```python
from build123d import *

# Parameters (mm, degrees)
SKETCH2_R           = 2
BOSS_EXTRUDE1_DEPTH = 14
SKETCH7_R           = 12.060749
CUT_EXTRUDE4_DEPTH  = 8
SKETCH8_R           = 2
CUT_EXTRUDE5_DEPTH  = 8
FILLET2_R           = 2
FILLET4_R           = 2
SKETCH10_R          = 4
BOSS_EXTRUDE3_DEPTH = 3
SKETCH13_R          = 4.000853
BOSS_EXTRUDE4_DEPTH = 3
SKETCH15_R          = 2.9
SKETCH15_R_2        = 1.5
BOSS_EXTRUDE5_DEPTH = 9
SKETCH16_R          = 2.9
SKETCH16_R_2        = 1.5
BOSS_EXTRUDE6_DEPTH = 9
CIRPATTERN1_COUNT   = 3


with BuildPart() as part:
    # Sketch2 → Boss-Extrude1 (new body)
    with BuildSketch(Plane.XY):
        with BuildLine():
            Line((-7, 23), (-7, 37))
            Line((-7, 37), (7, 37))
            Line((7, 37), (7, 23))
            ThreePointArc((7, 23), (13.037466, 7.527184), (23.418584, -5.437822))
            Line((23.418584, -5.437822), (35.54294, -12.437822))
            Line((35.54294, -12.437822), (28.54294, -24.562178))
            Line((28.54294, -24.562178), (16.418584, -17.562178))
            ThreePointArc((16.418584, -17.562178), (0, -15.054369), (-16.418584, -17.562178))
            Line((-16.418584, -17.562178), (-28.54294, -24.562178))
            Line((-28.54294, -24.562178), (-35.54294, -12.437822))
            Line((-35.54294, -12.437822), (-23.418584, -5.437822))
            ThreePointArc((-23.418584, -5.437822), (-13.037466, 7.527184), (-7, 23))
        make_face()
        Circle(SKETCH2_R, mode=Mode.SUBTRACT)
    extrude(amount=BOSS_EXTRUDE1_DEPTH)

    # Sketch7 → Cut-Extrude4 (cut)
    with BuildSketch(Plane.XY.offset(14)):
        Circle(SKETCH7_R)
    extrude(amount=-CUT_EXTRUDE4_DEPTH, mode=Mode.SUBTRACT)

    # Sketch8 → Cut-Extrude5 (cut)
    with BuildSketch(Plane.XY.offset(6)):
        with Locations((0, 8)):
            Circle(SKETCH8_R)
        with Locations((6.254652, 4.987918)):
            Circle(SKETCH8_R)
        with Locations((7.799423, -1.780167)):
            Circle(SKETCH8_R)
        with Locations((3.47107, -7.207751)):
            Circle(SKETCH8_R)
        with Locations((-3.47107, -7.207751)):
            Circle(SKETCH8_R)
        with Locations((-7.799423, -1.780167)):
            Circle(SKETCH8_R)
        with Locations((-6.254652, 4.987918)):
            Circle(SKETCH8_R)
    extrude(amount=-CUT_EXTRUDE5_DEPTH, mode=Mode.SUBTRACT)

    # Fillet2
    fillet2_edges = [part.edges().sort_by_distance(p)[0] for p in [
        (32.04294, -18.5, 0),
        (-32.04294, -18.5, 0),
        (0, 37, 0),
        (-32.04294, -18.5, 14),
        (32.04294, -18.5, 14),
        (0, 37, 14),
    ]]
    fillet(fillet2_edges, radius=FILLET2_R)

    # Fillet4
    fillet4_edges = [part.edges().sort_by_distance(p)[0] for p in [
        (7, 29, 0),
        (13.037466, 7.527184, 0),
        (-13.037466, 7.527184, 14),
        (21.614737, -20.562178, 0),
        (0, -15.054369, 0),
        (-28.614737, -8.437822, 0),
        (-13.037466, 7.527184, 0),
        (-28.614737, -8.437822, 14),
        (0, -15.054369, 14),
        (21.614737, -20.562178, 14),
        (13.037466, 7.527184, 14),
        (7, 29, 14),
        (-7, 37, 7),
        (7, 37, 7),
        (-7, 29, 0),
        (-7, 29, 14),
        (-7, 36.414214, 13.414214),
        (-7, 36.414214, 0.585786),
        (28.614737, -8.437822, 0),
        (-21.614737, -20.562178, 0),
        (7, 36.414214, 13.414214),
        (7, 36.414214, 0.585786),
        (-21.614737, -20.562178, 14),
        (28.614737, -8.437822, 14),
        (-28.54294, -24.562178, 7),
        (-35.54294, -12.437822, 7),
        (-28.035634, -24.269285, 13.414214),
        (-28.035634, -24.269285, 0.585786),
        (-35.035634, -12.144929, 13.414214),
        (-35.035634, -12.144929, 0.585786),
        (35.54294, -12.437822, 7),
        (28.54294, -24.562178, 7),
        (35.035634, -12.144929, 13.414214),
        (35.035634, -12.144929, 0.585786),
        (28.035634, -24.269285, 13.414214),
        (28.035634, -24.269285, 0.585786),
    ]]
    fillet(fillet4_edges, radius=FILLET4_R)

    # Sketch10 → Boss-Extrude3 (add)
    with BuildSketch(Plane(origin=(3.5, 6.062178, 0), x_dir=(0.866025403784439, -0.4999999999999995, 0), z_dir=(0.49999999999999944, 0.8660254037844389, 0))):
        with Locations((29.5, -7)):
            Circle(SKETCH10_R)
    boss_extrude3 = extrude(amount=BOSS_EXTRUDE3_DEPTH)

    # Sketch13 → Boss-Extrude4 (add)
    with BuildSketch(Plane(origin=(-3.5, -6.062178, 0), x_dir=(0.8660254037844386, -0.5, 0), z_dir=(-0.5000000000000001, -0.8660254037844387, 0))):
        with Locations(Location((29.5, 7, 0), (0, 0, 180))):
            Circle(SKETCH13_R)
    boss_extrude4 = extrude(amount=BOSS_EXTRUDE4_DEPTH)

    # Sketch15 → Boss-Extrude5 (add)
    with BuildSketch(Plane(origin=(5, 8.660254, 0), x_dir=(0.8660254037844389, -0.4999999999999997, 0), z_dir=(0.4999999999999997, 0.8660254037844389, 0))):
        with Locations(Location((29.5, -7, 0), (0, 0, 180))):
            Circle(SKETCH15_R)
        with Locations(Location((29.5, -7, 0), (0, 0, 180))):
            Circle(SKETCH15_R_2, mode=Mode.SUBTRACT)
    boss_extrude5 = extrude(amount=BOSS_EXTRUDE5_DEPTH)

    # Sketch16 → Boss-Extrude6 (add)
    with BuildSketch(Plane(origin=(-5, -8.660254, 0), x_dir=(0.8660254037844386, -0.4999999999999999, 0), z_dir=(-0.49999999999999994, -0.8660254037844387, 0))):
        with Locations(Location((29.5, 7, 0), (0, 0, 180))):
            Circle(SKETCH16_R)
        with Locations(Location((29.5, 7, 0), (0, 0, 180))):
            Circle(SKETCH16_R_2, mode=Mode.SUBTRACT)
    boss_extrude6 = extrude(amount=BOSS_EXTRUDE6_DEPTH)

    # CirPattern1: Boss-Extrude3, Boss-Extrude4, Boss-Extrude5, Boss-Extrude6 ×3 about axis
    cirpattern1_axis = Axis((0, 0, 0), (0, 0, 1))
    add([boss_extrude3.rotate(cirpattern1_axis, i * 360 / CIRPATTERN1_COUNT) for i in range(1, CIRPATTERN1_COUNT)])
    add([boss_extrude4.rotate(cirpattern1_axis, i * 360 / CIRPATTERN1_COUNT) for i in range(1, CIRPATTERN1_COUNT)])
    add([boss_extrude5.rotate(cirpattern1_axis, i * 360 / CIRPATTERN1_COUNT) for i in range(1, CIRPATTERN1_COUNT)])
    add([boss_extrude6.rotate(cirpattern1_axis, i * 360 / CIRPATTERN1_COUNT) for i in range(1, CIRPATTERN1_COUNT)])


solid = part.part
```
CAD build for the part. Positions are in the model's coordinates, mm. A direction names the side the tool comes from. Round coordinates to 2 decimals unless told otherwise and drop trailing zeros. Loops run counter-clockwise (first coordinate to the right, second up) from the corner with the lowest first, then second, coordinate; pieces in that order, holes last. Notation, with made-up numbers: M -2,8 L 27,8 A20 cw 27,38 Z; hole C 88.5,67.25 d10. An arc over 180 degrees is marked long. Return JSON: item names as keys, results as strings. Group by question number.
(1) Saw through at C-C, the plane y = -28. Give the number of separate pieces and of enclosed holes in the cut face, and give its area (3 significant figures).
(2) Drop flat-ended pins along their axis: P1, Ø3, axis at y = -2.5, z = 4.5, coming from the -X side; P2, Ø3.5, axis at x = 0, y = 0, coming from the +Z side; P3, Ø2.5, axis at y = 29.5, z = 5.5, coming from the +X side; P4, Ø2.5, axis at y = 29.5, z = 7, coming from the -X side. Give the stop position or say it passes through.
(3) Tool access for faces 1 (the cylindrical face through (8.479, 25.684, 5.798)), 2 (the flat face through (-15, -30.6, 5.8)), 3 (the cylindrical face through (21.895, -20.029, 13.43)), 4 (the cylindrical face through (-2.615, -11.774, 10.056)), 5 (the cylindrical face through (-6.43, 28.8, 13.4)): list every direction of +Z, -Z, +X, -X, +Y, -Y with a clear straight run to the whole face (end or side of a thin tool).
(4) Saw through at A-A, the plane x = 0. List the corners of the cut face in (y, z), and give its area (3 significant figures).
(5) Mould opens along Y. For faces 6 (the flat face through (19, 28, 8)), 7 (the cylindrical face through (34.748, -12.674, 7.07)), 8 (the cylindrical face through (31.5, -18.3, 0.6)) say: +Y half, -Y half, draft (parallel to the pull), parting line (faces both ways), or undercut.
(6) Wall check: probe 1 along Z at (x, y) = (-14.25, 29.5); probe 2 along Y at (x, z) = (-18.5, 6); probe 3 along X at (y, z) = (30, 6.25). Give the ranges that are in metal, low to high. Write a range as [from, to].
Answer list:
{
 "1": {"separate pieces": "2", "enclosed holes": "2", "area": "44.7 mm2"},
 "2": {"P1": "x = -36.14", "P2": "through", "P3": "x = 19", "P4": "x = -10"},
 "3": {"face 1": "+X", "face 2": "+Z, -Z, -Y", "face 3": "+Z, -Y", "face 4": "+Z", "face 5": "+Z, -X, +Y"},
 "4": {"outline": "M -15.05,2 A2 ccw -13.05,0 L -2,0 L -2,6 L -12.06,6 L -12.06,14 L -13.05,14 A2 ccw -15.05,12 Z; M 2,0 L 6,0 L 6,6 L 2,6 Z; M 10,0 L 35,0 A2 ccw 37,2 L 37,12 A2 ccw 35,14 L 12.06,14 L 12.06,6 L 10,6 Z", "area": "484 mm2"},
 "5": {"face 6": "draft", "face 7": "undercut", "face 8": "-Y half"},
 "6": {"probe 1": "[4.1, 5.5], [8.5, 9.9]", "probe 2": "[-32.4, -29.19], [-24.72, -19.21], [-18.76, -0.28], [26.78, 28.38], [30.62, 32.22]", "probe 3": "[-10, 10]"}
}
